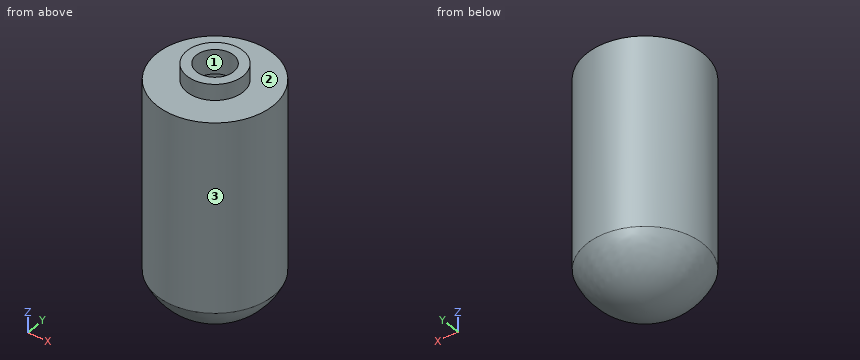
from build123d import *


with BuildPart() as f1:
    # F0 (on Front) → F1 (revolve)
    with BuildSketch(Plane.XZ):
        with BuildLine():
            Line((13.286673, 0), (0, 0))
            Line((0, 0), (0, -25.584204))
            ThreePointArc((0, -25.584204), (14.101099, -21.347377), (23.531822, -10.04016))
            Line((23.531822, -10.04016), (23.531822, 66.672839))
            Line((23.531822, 66.672839), (11.365706, 66.672839))
            Line((11.365706, 66.672839), (11.365706, 73.155217))
            Line((11.365706, 73.155217), (7.523784, 73.155217))
            Line((7.523784, 73.155217), (7.523784, 63.322656))
            Line((7.523784, 63.322656), (13.286673, 60.411584))
            Line((13.286673, 60.411584), (13.286673, 0))
        make_face()
    revolve(axis=Axis((0, 0, -12.792102), (0, 0, 1)))


solid = f1.part
Design review of the part built by this model. Coordinates are the model's own, in mm. Face numbers are marked on the shaded views. Give positions to 0.01 mm unless a question says otherwise; leave off trailing zeros. Loops run counter-clockwise (first coordinate to the right, second up) from the corner with the lowest first, then second, coordinate; pieces in that order, holes last. Notation, with made-up numbers: M 77,-13 L 100,-13 A23 ccw 100,24 Z; hole C -20,-35 d6. An arc over 180 degrees is marked long. Write item = value, one per line.
Q1. Draft analysis for pull direction Y (two halves, no side actions). For the marked faces 1, 2 and 3, state which applies: +Y half, -Y half, draft (parallel to the pull), parting line (faces both ways), or undercut.
Output values:
face_1 = undercut
face_2 = draft
face_3 = parting line
Q2. To check wall thickness, follow line 1 (Y direction, x = 0.5, z = 20); line 2 (Y direction, x = 0, z = 68); line 3 (X direction, y = 1, z = 25.5). State the ranges of each line that lie inside material, in increasing order. Write a range as [from, to].
Output values:
line_1 = [-23.53, -13.28], [13.28, 23.53]
line_2 = [-11.37, -7.52], [7.52, 11.37]
line_3 = [-23.51, -13.25], [13.25, 23.51]
Q3. Insertion check: pin 1 (4 mm diameter, centred on x = -18.5, y = 15.5, fed in from +Z); pin 2 (10 mm diameter, centred on x = -2, z = 58, fed in from +Y); pin 3 (3 mm diameter, centred on y = -2.5, z = 53.5, fed in from -X). Each pin has a flat end and moves straight along its axis. Give the tip position at first contact, or say it passes through.
Output values:
pin_1 = 66.67
pin_2 = 23.53
pin_3 = -23.51
Q4. We need section A-A (z = 47.5). Give the boundary of the cut face in (x, y).
Output values:
outline = C 0,0 d47.06; hole C 0,0 d26.57
